```python
from build123d import *

# Parameters (mm, degrees)
EXTRUDE_THIN1_DEPTH = 101.6
FILLET1_R           = 6.35
FILLET2_R           = 2.54
FILLET3_R           = 2.54
FILLET4_R           = 2.54
FILLET5_R           = 2.54
SKETCH4_W           = 137.085663299
SKETCH4_H           = 88.9
CUT_EXTRUDE1_DEPTH  = 20.32


# Read off the part's stored shape, not the designer's step: Extrude-Thin1
with BuildPart() as part:
    # Extrude-Thin1 outline → Extrude-Thin1 (new body)
    with BuildSketch(Plane.XY):
        Polygon((147.558789547, -4.59991125), (147.558789547, 15.496429633), (120.350988963, 20.80008875), (-18.530121413, 20.80008875), (-27.508924365, 10.64008875), (-58.181210453, 10.64008875), (-58.181210453, -4.59991125), align=None)
    extrude(amount=EXTRUDE_THIN1_DEPTH)

    # Fillet1
    fillet1_edges = [part.edges().sort_by_distance(p)[0] for p in [
        (-58.181210453, 10.64008875, 50.8),
    ]]
    fillet(fillet1_edges, radius=FILLET1_R)

    # Fillet2
    fillet2_edges = [part.edges().sort_by_distance(p)[0] for p in [
        (147.558789547, 15.496429633, 50.8),
    ]]
    fillet(fillet2_edges, radius=FILLET2_R)

    # Fillet3
    fillet3_edges = [part.edges().sort_by_distance(p)[0] for p in [
        (120.350988963, 20.80008875, 50.8),
        (-18.530121413, 20.80008875, 50.8),
    ]]
    fillet(fillet3_edges, radius=FILLET3_R)

    # Fillet4
    fillet4_edges = [part.edges().sort_by_distance(p)[0] for p in [
        (-27.508924365, 10.64008875, 50.8),
    ]]
    fillet(fillet4_edges, radius=FILLET4_R)

    # Fillet5
    fillet5_edges = [part.edges().sort_by_distance(p)[0] for p in [
        (-58.181210453, -0.15491125, 0),
        (-58.181210453, -0.15491125, 101.6),
        (-40.24258292, 10.64008875, 0),
        (-56.321338514, 8.780216811, 0),
        (-40.24258292, 10.64008875, 101.6),
        (-56.321338514, 8.780216811, 101.6),
        (147.558789547, 4.401918308, 0),
        (146.979144977, 15.018866002, 0),
        (147.558789547, 4.401918308, 101.6),
        (146.979144977, 15.018866002, 101.6),
        (133.048240824, 18.324993588, 0),
        (51.360321792, 20.80008875, 0),
        (120.349853607, 20.788330353, 0),
        (-18.428956215, 20.575675963, 0),
        (51.360321792, 20.80008875, 101.6),
        (133.048240824, 18.324993588, 101.6),
        (120.349853607, 20.788330353, 101.6),
        (-18.428956215, 20.575675963, 101.6),
        (-23.019522889, 15.72008875, 101.6),
        (-23.019522889, 15.72008875, 0),
        (-27.610089563, 10.864501537, 0),
        (-27.610089563, 10.864501537, 101.6),
    ]]
    fillet(fillet5_edges, radius=FILLET5_R)

    # Sketch4 → Cut-Extrude1 (cut)
    with BuildSketch(Plane(origin=(0, -4.59991125, 0), x_dir=(-1, 0, 0), z_dir=(0, -1, 0))):
        with Locations((-51.392828597, -50.8)):
            Rectangle(SKETCH4_W, SKETCH4_H)
    extrude(amount=-CUT_EXTRUDE1_DEPTH, mode=Mode.SUBTRACT)


solid = part.part
```
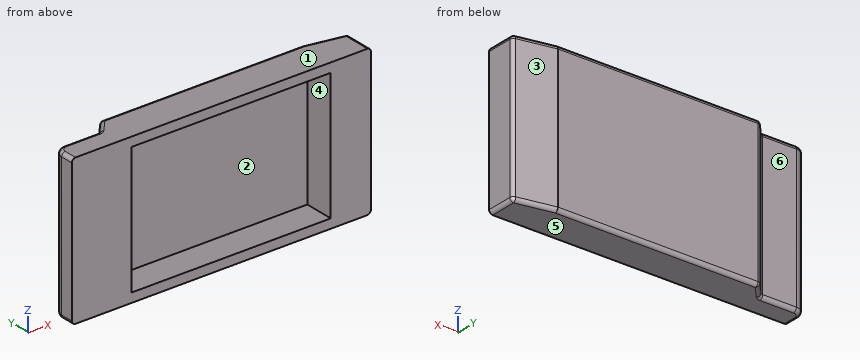
Build history of the part. All positions in model axes, mm. Face numbers are marked on the shaded views. A direction names the side the tool comes from. Round coordinates to 2 decimals unless told otherwise and drop trailing zeros. Write each loop counter-clockwise with the first axis right and the second up, starting at its lowest first coordinate (ties: lowest second). Pieces come first, ordered by that corner, then holes. Notation, with made-up numbers: (84.5, 79.5) - (113.5, 79.5) arc R25 cw to (113.5, 108.5) - close; hole circle Ø7 at (1.5, -23.75). An arc over 180 degrees is marked (long way). Write each question's results on one line, items separated by ' | '. Start each with the question number.
Item 1: Which spindle directions (+Z, -Z, +X, -X, +Y, -Y) get a long thin tool onto all of the face, cutting with end or side? Do the marked faces 4, 5 and 6. Say none if no direction does.
Item 2: Wall check: L1, parallel to X at y = -0.5, z = 36.5; L2, parallel to Z at x = 65, y = 7; L3, parallel to Y at x = 23.5, z = 61.5. Give the ranges that are in metal, low to high. Write a range as [from, to].
Item 3: Drop flat-ended pins along their axis: P1, Ø6, axis at x = 32, z = 40, coming from the -Y side; P2, Ø6, axis at y = 10.5, z = 72.5, coming from the -X side; P3, Ø11.5, axis at x = -42.5, z = 50.5, coming from the +Y side. Give the stop position or say it passes through.
Item 4: Mould opens along X. For the marked faces 1, 2 and 3 say: pulls with the +X half, pulls with the -X half, needs draft (parallel to the pull), parting line crosses it, or undercut.
Item 5: Saw through at A-A (y = 0.75). Write the cut outline in (x, z).
Item 6: Saw through at C-C (x = 1.5). Write the cut outline in (y, z).
Item 7: Saw through at B-B (z = 89). Write the cut outline in (x, y).
Results are:
1) face 4: -Y | face 5: -Z, +X, -X, +Y, -Y | face 6: +Z, -Z, -X, +Y
2) L1: x = [-58.18, -17.15], [119.94, 147.56] | L2: z = [0, 6.35], [95.25, 101.6] | L3: y = [15.72, 20.8]
3) P1: stops at y = 15.72 | P2: stops at x = -57.31 | P3: stops at y = 10.64
4) face 1: needs draft | face 2: undercut | face 3: pulls with the +X half
5) outline: (-58.18, 2.54) arc R2.54 ccw to (-55.64, 0) - (145.02, 0) arc R2.54 ccw to (147.56, 2.54) - (147.56, 99.06) arc R2.54 ccw to (145.02, 101.6) - (-55.64, 101.6) arc R2.54 ccw to (-58.18, 99.06) - close; hole (-17.15, 6.35) - (119.94, 6.35) - (119.94, 95.25) - (-17.15, 95.25) - close
6) outline: (-4.6, 0) - (18.26, 0) arc R2.54 ccw to (20.8, 2.54) - (20.8, 99.06) arc R2.54 ccw to (18.26, 101.6) - (-4.6, 101.6) - (-4.6, 95.25) - (15.72, 95.25) - (15.72, 6.35) - (-4.6, 6.35) - close
7) outline: (-58.18, -4.6) - (-17.15, -4.6) - (-17.15, 15.72) - (119.94, 15.72) - (119.94, -4.6) - (147.56, -4.6) - (147.56, 13.4) arc R2.54 ccw to (145.5, 15.9) - (120.59, 20.75) arc R2.54 ccw to (120.11, 20.8) - (-17.39, 20.8) arc R2.54 ccw to (-19.29, 19.94) - (-26.75, 11.5) arc R2.54 cw to (-28.65, 10.64) - (-51.83, 10.64) arc R6.35 ccw to (-58.18, 4.29) - close
